CAD build for the part. Positions are in the model's coordinates, mm. Coordinates: 2 decimals unless noted, no trailing zeros. Order: outer loops, then holes, each group sorted by start corner. A loop starts at its lowest first (then second) coordinate and runs counter-clockwise, first axis right, second up. Notation, with made-up numbers: M 41.25,85 L 94.25,85 A18 cw 94.25,106 Z; hole C -13.5,51 d8. An arc over 180 degrees is marked long. Write item = value, one per line.
Autodesk Inventor part; units mm, degrees
ref_plane "YZ Plane" through (0, 0, 0) normal (1, 0, 0) x (0, 1, 0)
ref_plane "XZ Plane" through (0, 0, 0) normal (0, 1, 0) x (-1, 0, 0)
ref_plane "XY Plane" through (0, 0, 0) normal (0, 0, 1) x (1, 0, 0)
sketch "Boceto1" plane through (0, 0, 0) normal (0, 1, 0) x (-1, 0, 0)
  line L0 (50, 100) -> (50, -100)
  line L1 (-50, 100) -> (50, -100) construction
  line L2 (50, 100) -> (-50, -100) construction
  line L3 (25, 100) -> (25, 97)
  line L4 (25, 97) -> (-25, 97)
  line L5 (-25, 97) -> (-25, 100)
  line L6 (-50, 100) -> (-25, 100)
  line L7 (25, 100) -> (50, 100)
  line L8 (25, -100) -> (25, -97)
  line L9 (25, -97) -> (-25, -97)
  line L10 (-25, -97) -> (-25, -100)
  line L11 (50, -100) -> (25, -100)
  line L12 (-25, -100) -> (-50, -100)
  line L13 (-50, -100) -> (-50, 100)
  point P0 (0, 0)
  dimension "d0" = 100
  dimension "d1" = 200
  dimension "d4" = 3
  dimension "d5" = 50
  dimension "d7" = 3
  dimension "d8" = 50
  dimension "d12" = 25
extrude "Extrusión1" add sketch "Boceto1" along normal blind 3
sketch "Boceto2" plane through (0, 3, 0) normal (0, 1, 0) x (1, 0, 0)
  line L0 (33, 12) -> (30, 12)
  line L1 (30, 12) -> (30, -38)
  line L2 (30, -38) -> (33, -38)
  line L3 (33, -38) -> (33, 12)
  line L4 (50, 100) -> (25, 100)
  line L5 (-50, 100) -> (-50, -100)
  point P0 (0, 0)
  dimension "d17" = 3
  dimension "d18" = 50
  dimension "d19" = 88
  dimension "d20" = 80
extrude "Extrusión2" cut sketch "Boceto2" against normal blind 3
sketch "Boceto3" plane through (0, 0, 0) normal (0, -1, 0) x (1, 0, 0)
  line L0 (-40, -1.5) -> (-10, -1.5)
  line L1 (-10, -1.5) -> (-10, 1.5)
  line L2 (-10, 1.5) -> (-40, 1.5)
  line L3 (-40, 1.5) -> (-40, -1.5)
  line L4 (-50, -100) -> (-25, -100)
  line L5 (30, -12) -> (30, 38)
  point P0 (0, 0)
  dimension "d23" = 30
  dimension "d24" = 3
  dimension "d25" = 98.5
  dimension "d26" = 40
extrude "Extrusión3" cut sketch "Boceto3" against normal blind 3
sketch "Boceto4" plane through (0, 3, 0) normal (0, 1, 0) x (1, 0, 0)
  line L0 (28, 1.5) -> (20, 1.5)
  line L1 (20, 1.5) -> (20, -53.5)
  line L2 (20, -53.5) -> (28, -53.5)
  line L3 (28, -53.5) -> (28, 1.5)
  line L4 (-25, -97) -> (25, -97)
  line L5 (30, -38) -> (30, 12)
  line L6 (28, -26) -> (20, -26) construction
  line L7 (25, -100) -> (50, -100)
  point P0 (0, 0)
  dimension "d29" = 55
  dimension "d30" = 8
  dimension "d32" = 2
  dimension "d35" = 74
extrude "Extrusión4" cut sketch "Boceto4" against normal blind 3
properties part number "Piso"
(1) Pin check, flat tips, straight feed: pin 1 Ø0.9 at (x, y) = (5, 1.5) entering from -Z; pin 2 Ø6 at (x, z) = (-22, 6) entering from -Y; pin 3 Ø0.9 at (x, y) = (24, 1.5) entering from +Z. Stop position of each tip, or through.
Evaluation:
pin_1 = -97
pin_2 = 0
pin_3 = 97
(2) Wall check: line 1 (X direction, y = 0.25, z = 13); line 2 (Z direction, x = 21, y = 0.5); line 3 (X direction, y = 0.4, z = -9). Give the ranges that are in metal, low to high. Write a range as from..to.
Evaluation:
line_1 = -50..20, 28..30, 33..50
line_2 = -97..-1.5, 53.5..97
line_3 = -50..30, 33..50
(3) Slice it at A-A, the plane z = 34. Write the cut outline in (x, y), then the cut area to 3 significant figures.
Evaluation:
outline = M -50,0 L 20,0 L 20,3 L -50,3 Z; M 28,0 L 30,0 L 30,3 L 28,3 Z; M 33,0 L 50,0 L 50,3 L 33,3 Z
area = 267 mm²
(4) Slice it at D-D, the plane x = -19.5. Write the cut outline in (y, z).
Evaluation:
outline = M 0,-97 L 3,-97 L 3,-1.5 L 0,-1.5 Z; M 0,1.5 L 3,1.5 L 3,97 L 0,97 Z
(5) Slice it at B-B, the plane x = -29.5. Write the cut outline in (y, z), then the cut area to 3 significant figures.
Evaluation:
outline = M 0,-100 L 3,-100 L 3,-1.5 L 0,-1.5 Z; M 0,1.5 L 3,1.5 L 3,100 L 0,100 Z
area = 591 mm²
(6) Slice it at C-C, the plane y = 1.8. Write the cut outline in (x, z), then the cut area to 3 significant figures.
Evaluation:
outline = M -50,-100 L -25,-100 L -25,-97 L 25,-97 L 25,-100 L 50,-100 L 50,100 L 25,100 L 25,97 L -25,97 L -25,100 L -50,100 Z; hole M -40,-1.5 L -10,-1.5 L -10,1.5 L -40,1.5 Z; hole M 20,-1.5 L 28,-1.5 L 28,53.5 L 20,53.5 Z; hole M 30,-12 L 33,-12 L 33,38 L 30,38 Z
area = 19,000 mm²
